Read the model definition and answer for the solid it produces. Units are mm, in the model's axes. A direction names the side the tool comes from. Give positions to 0.01 mm unless a question says otherwise; leave off trailing zeros. Loops run counter-clockwise (first coordinate to the right, second up) from the corner with the lowest first, then second, coordinate; pieces in that order, holes last.
(1) Find section D-D, the plane y = -34.5. Write down the section's boundary in (x, z), then the cut area to 3 significant figures.
(2) Find section A-A, the plane z = 9. Write down the section's boundary in (x, y).
(3) Which of the six approach directions +Z, -Z, +X, -X, +Y, -Y give full straight-line access (tool end or side, diameter ignored) to faces 1 (the face through (-22, -19, 25.4)), 2 (the face through (0, -25.4, 13)), 3 (the face through (-50.251, -38, 13)), 4 (the face through (-13, -19, 0)), 5 (the face through (-25.4, -13, -13))?
(4) Find section B-B, the plane y = -5.5. Write down the section's boundary in (x, z).
(5) Find section C-C, the plane x = -46. Write down the section's boundary in (y, z).
(6) Each of these flat-tipped pins is pushed along its axis until it touches: P1, Ø12.5, axis at y = -8.5, z = -8, coming from the +X side; P2, Ø7.5, axis at x = -11, z = 6.5, coming from the -Y side; P3, Ø12.5, axis at y = -42, z = 10.5, coming from the +X side. Where does it stop, or does it pass through?
(7) Straight lines are drawn through the part: probe 1 along Z at (x, y) = (-33.5, -34.5); probe 2 along Y at (x, z) = (-44, -12.5); probe 3 along X at (y, z) = (-2.5, -20). For each, find the intervals that lie inside material, in ascending order.
```python
from build123d import *

# Parameters (mm, degrees)
F0_W     = 25.4
F0_H     = 25.4
F1_DEPTH = 25.4
F2_W     = 25.4
F2_H     = 25.4
F3_DEPTH = 25.4


with BuildPart() as f1:
    # F0 (on Front) → F1 (new body)
    with BuildSketch(Plane.XZ):
        with Locations((-38.1, 12.7)):
            Rectangle(F0_W, F0_H)
        with Locations((-38.1, -12.7)):
            Rectangle(F0_W, F0_H)
        with Locations((-12.7, 12.7)):
            Rectangle(F0_W, F0_H)
        with Locations((12.7, 12.7)):
            Rectangle(F0_W, F0_H)
    extrude(amount=F1_DEPTH)

    # F2 (on Top) → F3 (join)
    with BuildSketch(Plane.XY):
        with Locations((-37.550894, -37.707685)):
            Rectangle(F2_W, F2_H)
    extrude(amount=F3_DEPTH)


solid = f1.part
```
Entries:
1. outline: (-50.25, 0) - (-24.85, 0) - (-24.85, 25.4) - (-50.25, 25.4) - close
1. area: 645 mm2
2. outline: (-50.8, -25.4) - (-50.25, -25.4) - (-50.25, -50.41) - (-24.85, -50.41) - (-24.85, -25.4) - (25.4, -25.4) - (25.4, 0) - (-50.8, 0) - close
3. face 1: +Z, +X, -X, +Y, -Y
3. face 2: +Z, -Z, +X, -Y
3. face 3: +Z, -Z, -X, -Y
3. face 4: -Z, +X, -Y
3. face 5: -Z, +X, +Y, -Y
4. outline: (-50.8, -25.4) - (-25.4, -25.4) - (-25.4, 0) - (25.4, 0) - (25.4, 25.4) - (-50.8, 25.4) - close
5. outline: (-50.41, 0) - (-25.4, 0) - (-25.4, -25.4) - (0, -25.4) - (0, 25.4) - (-50.41, 25.4) - close
6. P1: stops at x = -25.4
6. P2: stops at y = -25.4
6. P3: stops at x = -24.85
7. probe 1: z = 0 to 25.4
7. probe 2: y = -25.4 to 0
7. probe 3: x = -50.8 to -25.4
